Verification items for the finished model (mm, model axes). A direction names the side the tool comes from. Round coordinates to 2 decimals unless told otherwise and drop trailing zeros. Order: outer loops, then holes, each group sorted by start corner. A loop starts at its lowest first (then second) coordinate and runs counter-clockwise, first axis right, second up. Notation, with made-up numbers: (61, 67.5) -> (69, 67.5) arc R17 cw to (69, 72.5) -> close; hole circle Ø7 at (-39.5, -28.75). An arc over 180 degrees is marked (long way). Put each result on its own line as item: value.
from build123d import *

# Parameters (mm, degrees)
F0_R     = 1.25
F1_DEPTH = 10
F2_R     = 2
F3_DEPTH = 13.501
F4_R     = 1


# Not quite as in the source:
# - a feature names something its author has since deleted; it is built from what else it names


with BuildPart() as f1:
    # F0 (on Top) → F1 (new body)
    with BuildSketch(Plane.XY):
        Polygon((2.875, 0), (-2.875, 0), (-2.875, -1.5), (-9.875, -1.5), (-9.875, -13.5), (5.875, -13.5), (5.875, -1.5), (2.875, -1.5), align=None)
        with Locations((-6, -10)):
            Circle(F0_R, mode=Mode.SUBTRACT)
    extrude(amount=F1_DEPTH)

    # F2 (on face) → F3 (cut, through all)
    with BuildSketch(Plane.XZ.offset(13.5)):
        with Locations((0, 5)):
            Circle(F2_R)
    extrude(amount=-F3_DEPTH, mode=Mode.SUBTRACT)

    # F4
    f4_edges = [f1.edges().sort_by_distance(p)[0] for p in [
        (5.875, -1.5, 5),
        (5.875, -13.5, 5),
        (-9.875, -1.5, 5),
        (-9.875, -13.5, 5),
    ]]
    fillet(f4_edges, radius=F4_R)


solid = f1.part
Item 1: Section check D-D on z = 2.75. Record the boundary of the cut face in (x, y) (3 decimals).
Check sheet entries:
outline: (-9.875, -12.5) arc R1 ccw to (-8.875, -13.5) -> (4.875, -13.5) arc R1 ccw to (5.875, -12.5) -> (5.875, -2.5) arc R1 ccw to (4.875, -1.5) -> (2.875, -1.5) -> (2.875, 0) -> (-2.875, 0) -> (-2.875, -1.5) -> (-8.875, -1.5) arc R1 ccw to (-9.875, -2.5) -> close; hole circle Ø2.5 at (-6, -10)
Item 2: Section check A-A on y = -10. Record the boundary of the cut face in (x, z) (3 decimals), then the cut area to 3 significant figures.
Check sheet entries:
outline: (-9.875, 0) -> (-7.25, 0) -> (-7.25, 10) -> (-9.875, 10) -> close; (-4.75, 0) -> (5.875, 0) -> (5.875, 10) -> (-4.75, 10) -> close; hole circle Ø4 at (0, 5)
area: 120 mm^2
Item 3: Section check B-B on z = 5. Record the boundary of the cut face in (x, y) (3 decimals).
Check sheet entries:
outline: (-9.875, -12.5) arc R1 ccw to (-8.875, -13.5) -> (-2, -13.5) -> (-2, 0) -> (-2.875, 0) -> (-2.875, -1.5) -> (-8.875, -1.5) arc R1 ccw to (-9.875, -2.5) -> close; (2, -13.5) -> (4.875, -13.5) arc R1 ccw to (5.875, -12.5) -> (5.875, -2.5) arc R1 ccw to (4.875, -1.5) -> (2.875, -1.5) -> (2.875, 0) -> (2, 0) -> close; hole circle Ø2.5 at (-6, -10)
Item 4: Material ranges on L1, parallel to Z at x = 0, y = -10.5; L2, parallel to Y at x = -6, z = 6; L3, parallel to Y at x = -3.75, z = 4, recorded low to high. Write a range as [from, to].
Check sheet entries:
L1: z = [0, 3], [7, 10]
L2: y = [-13.5, -11.25], [-8.75, -1.5]
L3: y = [-13.5, -1.5]
Item 5: Section check C-C on x = 0. Record the boundary of the cut face in (y, z).
Check sheet entries:
outline: (-13.5, 0) -> (0, 0) -> (0, 3) -> (-13.5, 3) -> close; (-13.5, 7) -> (0, 7) -> (0, 10) -> (-13.5, 10) -> close
Item 6: Tool access check on faces 1 (the flat face through (-9.875, -7, 5)), 2 (the flat face through (-2.875, -1, 5)), 3 (the flat face through (2.875, -1, 5)). Record the directions out of +Z, -Z, +X, -X, +Y, -Y that give a thin tool (end or side, any length) a straight path to the whole face; none if there is none.
Check sheet entries:
face 1: +Z, -Z, -X, +Y, -Y
face 2: +Z, -Z, -X, +Y
face 3: +Z, -Z, +X, +Y
Item 7: Release check for a two-part mould opening along Y. For faces 4 (the flat face through (-2, -13.5, 4)), 5 (the flat face through (2, 0, 4)), 6 (the cylindrical face through (-6.921, -9.155, 4.93)) record: +Y half, -Y half, draft (parallel to the pull), parting line (faces both ways), or undercut.
Check sheet entries:
face 4: -Y half
face 5: +Y half
face 6: undercut
Item 8: Gauge pin test, flat ends, axial feed: pin 1 Ø1.6 at (y, z) = (-1, 6) entering from +X; pin 2 Ø1.8 at (x, z) = (-6, 6) entering from +Y; pin 3 Ø3 at (x, z) = (0, 5) entering from +Y; pin 4 Ø0.8 at (y, z) = (-1, 6.5) entering from -X (3 decimals). Record the tip position at first contact, or that the pin passes through.
Check sheet entries:
pin 1: stops at x = 5.59
pin 2: stops at y = -1.5
pin 3: passes through
pin 4: stops at x = -2.875
